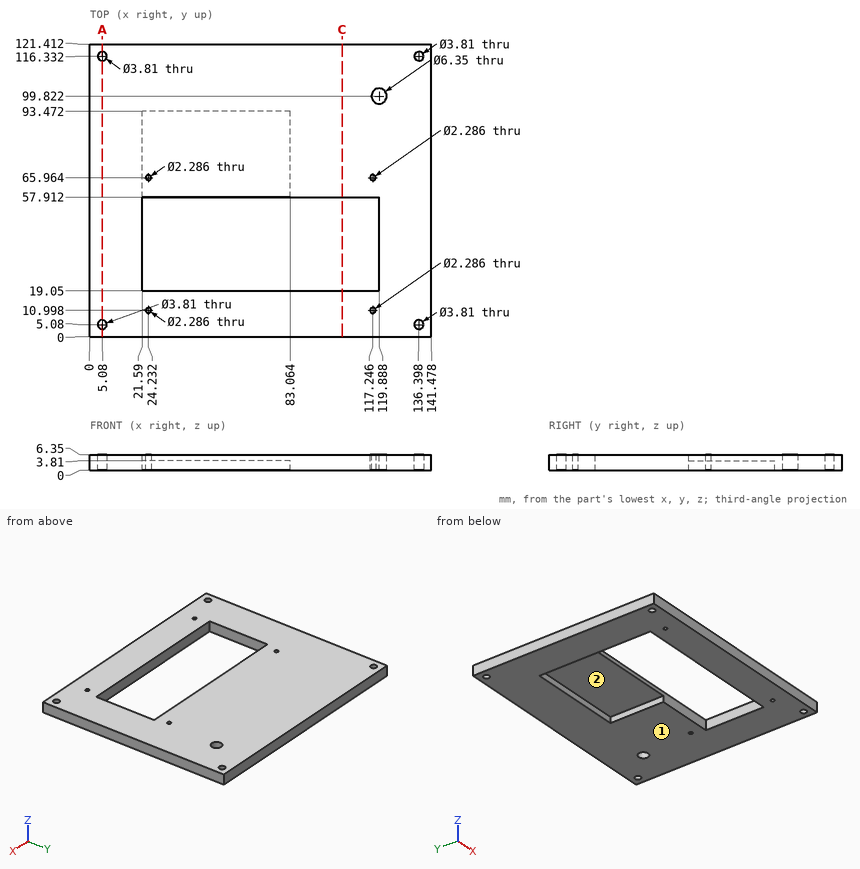
Design review of the part shown in the three views and the two pictorial views. Dimensions are in mm from the part's minimum x, y and z. Give positions to 0.01 mm unless a question says otherwise; leave off trailing zeros. Write each loop counter-clockwise with the first axis right and the second up, starting at its lowest first coordinate (ties: lowest second). Pieces come first, ordered by that corner, then holes. Notation, with made-up numbers: M 63.5,-25.75 L 121.5,-25.75 A29 ccw 121.5,3.25 Z; hole C 84,86 d11. An arc over 180 degrees is marked long. One line per question, with ' | ' between items. Start each with the question number.
Item 1: We need section A-A on x = 5.08. Give the number of separate pieces and of enclosed holes in the cut face.
Item 2: We need section C-C on x = 104.5. Write out the cut boundary in (y, z), plus the area to 3 significant figures.
Item 3: Draft analysis for pull direction Y (two halves, no side actions). For the marked faces 1 and 2, state which applies: released by +Y, released by -Y, zero draft, split by the parting line, or undercut.
Item 4: For pin 1 (4 mm diameter, centred on x = 119.888, y = 99.822, fed in from -Z); pin 2 (2.5 mm diameter, centred on x = 24.23, y = 65.96, fed in from -Z), all flat-tipped, find the tip position at first contact; note any pin that passes through.
Item 5: Wall thickness on line 1 (Y direction, x = 24, z = 0.75); line 2 (X direction, y = 28.5, z = 2); line 3 (X direction, y = 71.5, z = 3): over which ranges is each line inside the solid? List them lowest first. Write a range as from..to.
Results found:
1) separate pieces: 3 | enclosed holes: 0
2) outline: M 0,0 L 19.05,0 L 19.05,6.35 L 0,6.35 Z; M 57.91,0 L 121.41,0 L 121.41,6.35 L 57.91,6.35 Z | area: 524 mm2
3) face 1: zero draft | face 2: undercut
4) pin 1: passes through | pin 2: stops at z = 3.81
5) line 1: y = 0..9.88, 12.12..19.05, 93.47..121.41 | line 2: x = 0..21.59, 119.89..141.48 | line 3: x = 0..21.59, 83.06..141.48
